Source: three-view drawing plus pictorial views. Frame: mm from the lowest corner of the part. Round coordinates to 2 decimals unless told otherwise and drop trailing zeros. Order: outer loops, then holes, each group sorted by start corner. A loop starts at its lowest first (then second) coordinate and runs counter-clockwise, first axis right, second up. Notation, with made-up numbers: M -38.75,45.25 L -32.75,45.25 A21 ccw -32.75,56.25 Z; hole C -35.5,9.5 d7. An arc over 180 degrees is marked long. Return JSON: item names as keys, results as strings. Group by question number.
Q1. Cut plane A-A on z = 42.5. Output: boundary loops of the cut face in (x, y).
Q2. Contact query for flat-ended pins moving along their axis: pin 1 (3 mm diameter, centred on x = 26, z = 69.5, fed in from +Y); pin 2 (4 mm diameter, centred on x = 299.5, z = 60, fed in from +Y); pin 3 (5 mm diameter, centred on x = 1146, y = 40.5, fed in from +Z). Output: stop coordinate, or through.
Q3. Ray query, probe 1 along X at (y, z) = (15.5, 60); probe 2 along Y at (x, z) = (295.5, 43); probe 3 along Y at (x, z) = (263, 46). Return the intervals inside material, ascending.
Q4. Cut plane B-B on x = 410. Output: boundary loops of the cut face in (y, z).
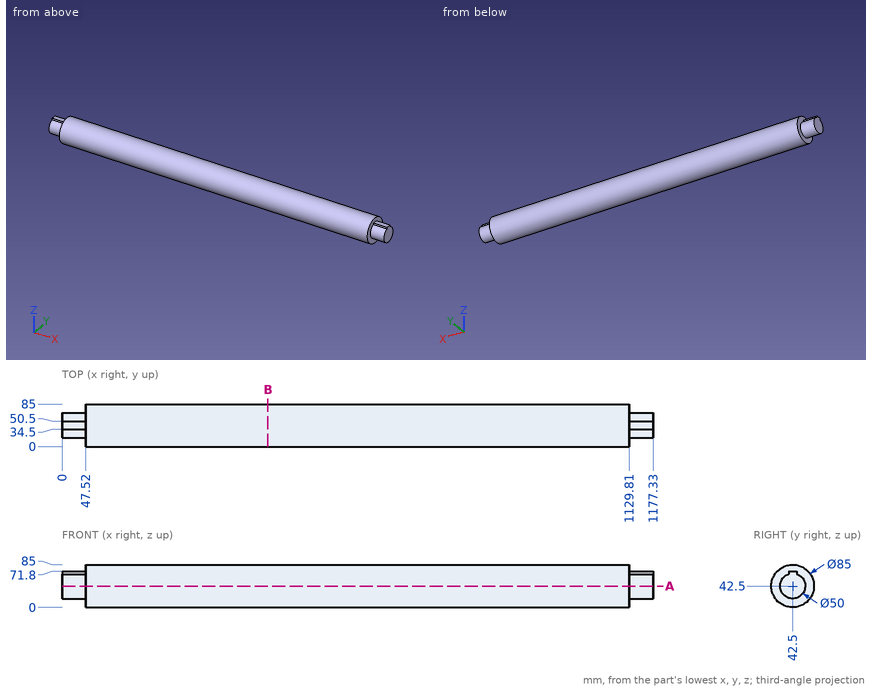
Result sheet:
{
 "1": {"outline": "M 0,17.5 L 47.52,17.5 L 47.52,0 L 1129.81,0 L 1129.81,17.5 L 1177.33,17.5 L 1177.33,67.5 L 1129.81,67.5 L 1129.81,85 L 47.52,85 L 47.52,67.5 L 0,67.5 Z"},
 "2": {"pin 1": "stops at y = 50.5", "pin 2": "stops at y = 82.07", "pin 3": "stops at z = 71.8"},
 "3": {"probe 1": "x = 47.52 to 1129.81", "probe 2": "y = 0 to 85", "probe 3": "y = 0.14 to 84.86"},
 "4": {"outline": "C 42.5,42.5 d85"}
}
